Model file for the job. Use its own axes, mm. A direction names the side the tool comes from. Give positions to 0.01 mm unless a question says otherwise; leave off trailing zeros. Order: outer loops, then holes, each group sorted by start corner. A loop starts at its lowest first (then second) coordinate and runs counter-clockwise, first axis right, second up. Notation, with made-up numbers: M 34,46 L 61,46 A9 ccw 61,61 Z; hole C 41.25,-36 d7. An arc over 180 degrees is marked long. Return JSON: item names as keys, results as strings. Group by question number.
1. Slice it at A-A on z = 1.45. List the corners of the cut face in (x, y), then the cut area to 3 significant figures.
2. Two-plate mould, pull along X, no slides. Class faces 5 (the face through (3, 45, 3)), 6 (the face through (0, 53, 3)), 7 (the face through (50, 3, 3)): released by +X, released by -X, zero draft, split by the parting line, or undercut.
3. Wall check: probe 1 along Y at (x, z) = (51, 0.7); probe 2 along X at (y, z) = (25, 0.25). Give the ranges that are in metal, low to high. Write a range as [from, to].
4. Slice it at C-C on y = 29.5. List the corners of the cut face in (x, z).
5. Slice it at B-B on x = 71.5. List the corners of the cut face in (y, z), then the cut area to 3 significant figures.
6. 3-axis set-ups, long thin cutter, end or side, ignore diameter. For faces 1 (the face through (3, 15, 3)), 2 (the face through (189, 15, 3)), 3 (the face through (95, 5.2, 3)), 4 (the face through (25, 0, 3)): which of +Z, -Z, +X, -X, +Y, -Y reach the whole face in a straight line?
Autodesk Inventor part; units mm, degrees
ref_plane "YZ Plane" through (0, 0, 0) normal (1, 0, 0) x (0, 1, 0)
ref_plane "XZ Plane" through (0, 0, 0) normal (0, 1, 0) x (-1, 0, 0)
ref_plane "XY Plane" through (0, 0, 0) normal (0, 0, 1) x (1, 0, 0)
sketch "Sketch1" plane through (0, 0, 0) normal (0, 0, 1) x (1, 0, 0)
  line L0 (0, 0) -> (192, 0)
  line L1 (192, 0) -> (192, 60)
  line L2 (192, 60) -> (0, 60)
  line L3 (0, 60) -> (0, 0)
  line L4 (192, 45) -> (186.8, 45)
  line L5 (186.8, 45) -> (186.8, 15)
  line L6 (186.8, 15) -> (192, 15)
  line L7 (192, 15) -> (192, 45)
  line L8 (0, 45) -> (5.2, 45)
  line L9 (5.2, 45) -> (5.2, 15)
  line L10 (5.2, 15) -> (0, 15)
  line L11 (0, 15) -> (0, 45)
  line L12 (142, 0) -> (50, 0)
  line L13 (50, 0) -> (50, 5.2)
  line L14 (50, 5.2) -> (142, 5.2)
  line L15 (142, 5.2) -> (142, 0)
  dimension "d0" = 60
  dimension "d1" = 192
  dimension "d4" = 5.2
  dimension "d5" = 30
  dimension "d6" = 15
  dimension "d7" = 30
  dimension "d8" = 5.2
  dimension "d9" = 15
  dimension "d12" = 50
  dimension "d13" = 50
  dimension "d14" = 5.2
extrude "Extrusion3" add sketch "Sketch1" along normal blind 5.2 contours L3 L10 L9 L8 L2 L1 L4 L5 L6 L0 L15 L14 L13
properties part number "Back Plate"
Result:
{
 "1": {"outline": "M 0,0 L 50,0 L 50,5.2 L 142,5.2 L 142,0 L 192,0 L 192,15 L 186.8,15 L 186.8,45 L 192,45 L 192,60 L 0,60 L 0,45 L 5.2,45 L 5.2,15 L 0,15 Z", "area": "10,700 mm2"},
 "2": {"face 5": "zero draft", "face 6": "released by -X", "face 7": "undercut"},
 "3": {"probe 1": "y = [5.2, 60]", "probe 2": "x = [5.2, 186.8]"},
 "4": {"outline": "M 5.2,0 L 186.8,0 L 186.8,5.2 L 5.2,5.2 Z"},
 "5": {"outline": "M 5.2,0 L 60,0 L 60,5.2 L 5.2,5.2 Z", "area": "285 mm2"},
 "6": {"face 1": "+Z, -Z, -X", "face 2": "+Z, -Z, +X", "face 3": "+Z, -Z, -Y", "face 4": "+Z, -Z, +X, -X, -Y"}
}
